Geometry check sheet. Reference: the model listing, model coordinates, mm. A direction names the side the tool comes from. Coordinates: 2 decimals unless noted, no trailing zeros. Write each loop counter-clockwise with the first axis right and the second up, starting at its lowest first coordinate (ties: lowest second). Pieces come first, ordered by that corner, then holes. Notation, with made-up numbers: M 52,-19 L 86,-19 A10 cw 86,-7 Z; hole C 53.5,75.25 d11. An arc over 180 degrees is marked long. Put each result on its own line as item: value. Start each with the question number.
1) Cross-section at C-C on z = -1.5. Record the cut outline in (x, y).
2) Scan lines: line 1 along Y through (x, z) = (0, -2.5); line 2 along Y through (x, z) = (0, -8); line 3 along X through (y, z) = (7, -6.25) (1 decimal). Record each from-to range of solid material in increasing order.
3) Gauge pin test, flat ends, axial feed: pin 1 (0.6 mm diameter, centred on x = 14, y = -7.5, fed in from +Z); pin 2 (10 mm diameter, centred on x = 0, y = 0, fed in from -Z); pin 3 (1.5 mm diameter, centred on x = 5.5, z = -7, fed in from +Y). Record the tip position at first contact, or that the pin passes through.
4) Cross-section at D-D on z = -22. Record the cut outline in (x, y), plus the area to 3 significant figures.
5) Cross-section at B-B on y = 0. Record the cut outline in (x, z), plus the area to 3 significant figures.
6) Set-up check for faces 3 (the flat face through (0, 0, -20)), 4 (the flat face through (16, -2, -5.5)): record each of +Z, -Z, +X, -X, +Y, -Y from which the full face is reachable in a straight line by a thin tool's end or side.
7) Mould release check, pull along Y, two halves, no side actions. Record for faces 1 (the flat face through (0, -18, 0)), 2 (the flat face through (-3, -16, -5.5)): released by +Y, released by -Y, zero draft, split by the parting line, or undercut.
8) Cross-section at A-A on z = -8.75. Count the separate pieces of the cut face and the enclosed holes in it, plus the area to 3 significant figures.
from build123d import *

# Parameters (mm, degrees)
SKETCH1_R           = 20
BOSS_EXTRUDE1_DEPTH = 25
SKETCH2_R           = 17.5
SKETCH2_R_2         = 15
CUT_EXTRUDE1_DEPTH  = 10
SKETCH3_R           = 4.4
CUT_EXTRUDE2_DEPTH  = 7
SKETCH4_R           = 12.5
CUT_EXTRUDE3_DEPTH  = 5
SKETCH5_R           = 1
BOSS_EXTRUDE2_DEPTH = 4.5


with BuildPart() as part:
    # Sketch1 → Boss-Extrude1 (new body)
    with BuildSketch(Plane.XY):
        Circle(SKETCH1_R)
    extrude(amount=-BOSS_EXTRUDE1_DEPTH)

    # Sketch2 → Cut-Extrude1 (cut)
    with BuildSketch(Plane.XY):
        Circle(SKETCH2_R)
        Circle(SKETCH2_R_2, mode=Mode.SUBTRACT)
    extrude(amount=-CUT_EXTRUDE1_DEPTH, mode=Mode.SUBTRACT)

    # Sketch3 → Cut-Extrude2 (cut)
    with BuildSketch(Plane.XY):
        Circle(SKETCH3_R)
    extrude(amount=-CUT_EXTRUDE2_DEPTH, mode=Mode.SUBTRACT)

    # Sketch4 → Cut-Extrude3 (cut)
    with BuildSketch(Plane(origin=(0, 0, -25), x_dir=(-1, 0, 0), z_dir=(0, 0, -1))):
        Circle(SKETCH4_R)
    extrude(amount=-CUT_EXTRUDE3_DEPTH, mode=Mode.SUBTRACT)

    # Sketch5 → Boss-Extrude2 (add)
    with BuildSketch(Plane.XY.offset(-10)):
        with Locations((0, 16.25)):
            Circle(SKETCH5_R)
        with Locations((6.60947045, 14.845113687)):
            Circle(SKETCH5_R)
        with Locations((12.076103414, 10.873372353)):
            Circle(SKETCH5_R)
        with Locations((15.45466839, 5.021526159)):
            Circle(SKETCH5_R)
        with Locations((16.1609808, -1.698587528)):
            Circle(SKETCH5_R)
        with Locations((14.072912811, -8.125)):
            Circle(SKETCH5_R)
        with Locations((9.55151035, -13.146526159)):
            Circle(SKETCH5_R)
        with Locations((3.378564976, -15.894898512)):
            Circle(SKETCH5_R)
        with Locations((-3.378564976, -15.894898512)):
            Circle(SKETCH5_R)
        with Locations((-9.55151035, -13.146526159)):
            Circle(SKETCH5_R)
        with Locations((-14.072912811, -8.125)):
            Circle(SKETCH5_R)
        with Locations((-16.1609808, -1.698587528)):
            Circle(SKETCH5_R)
        with Locations((-15.45466839, 5.021526159)):
            Circle(SKETCH5_R)
        with Locations((-12.076103414, 10.873372353)):
            Circle(SKETCH5_R)
        with Locations((-6.60947045, 14.845113687)):
            Circle(SKETCH5_R)
    extrude(amount=BOSS_EXTRUDE2_DEPTH)


solid = part.part
Answer key:
1. outline: C 0,0 d40; C 0,0 d30; hole C 0,0 d35; hole C 0,0 d8.8
2. line 1: y = -20 to -17.5, -15 to -4.4, 4.4 to 15, 17.5 to 20
2. line 2: y = -20 to -17.5, -15 to 15, 15.25 to 17.25, 17.5 to 20
2. line 3: x = -18.7 to -16, -13.3 to 13.3, 16 to 18.7
3. pin 1: stops at z = -5.5
3. pin 2: stops at z = -20
3. pin 3: stops at y = 19.43
4. outline: C 0,0 d40; hole C 0,0 d25
4. area: 766 mm²
5. outline: M -20,-25 L -12.5,-25 L -12.5,-20 L 12.5,-20 L 12.5,-25 L 20,-25 L 20,0 L 17.5,0 L 17.5,-10 L 15,-10 L 15,0 L 4.4,0 L 4.4,-7 L -4.4,-7 L -4.4,0 L -15,0 L -15,-10 L -17.5,-10 L -17.5,0 L -20,0 Z
5. area: 763 mm²
6. face 3: -Z
6. face 4: +Z
7. face 1: zero draft
7. face 2: undercut
8. separate pieces: 17
8. enclosed holes: 1
8. area: 1,050 mm²
